Geometry: see drawing. Coordinates: mm, zero at the bounding-box minimum. A direction names the side the tool comes from. Give positions to 0.01 mm unless a question says otherwise; leave off trailing zeros. Order: outer loops, then holes, each group sorted by start corner. A loop starts at its lowest first (then second) coordinate and runs counter-clockwise, first axis right, second up. Notation, with made-up numbers: (-26, 27) - (-6, 27) arc R22 ccw to (-6, 58) - close; hole circle Ø4 at (25.25, 54.25). An arc over 180 degrees is marked (long way). Write item = value, one per line. Start each with the question number.
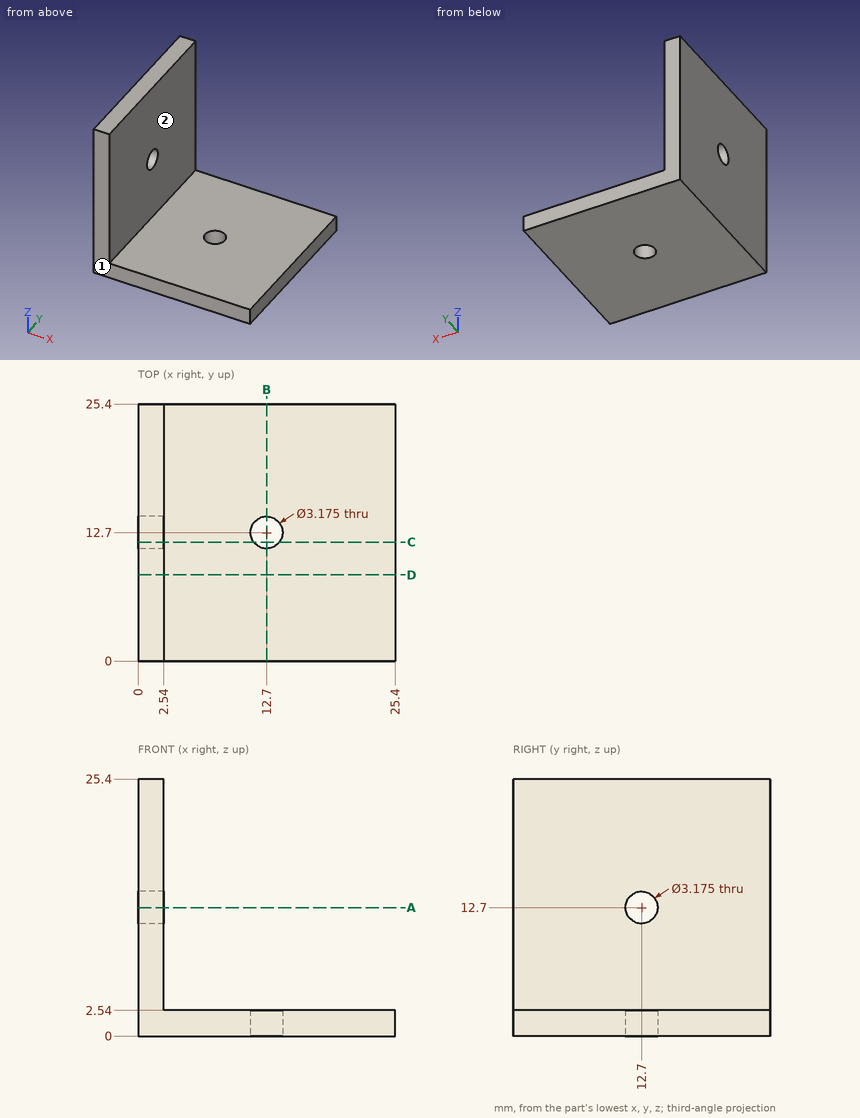
Q1. Section D-D, the plane y = 8.5. Return the cut outline in (x, z), then the cut area to 3 significant figures.
Q2. Section C-C, the plane y = 11.75. Return the cut outline in (x, z), then the cut area to 3 significant figures.
Q3. Set-up query: the marked faces 1 and 2. Return all of +Z, -Z, +X, -X, +Y, -Y with unobstructed straight access to the full face (end or side cutting, diameter ignored); none if empty.
Q4. Section A-A, the plane z = 12.7. Return the cut outline in (x, y).
Q5. Section B-B, the plane x = 12.7. Return the cut outline in (y, z).
Q6. Contact query for a flat-ended pin moving along its axis: pin 1 (8 mm diameter, centred on y = 6, z = 21.5, fed in from +X). Output: stop coordinate, or through.
Q7. Material intervals for line 1 along X through (y, z) = (8, 12.25); line 2 along Y through (x, z) = (12.7, 2), sorted ascending. Write a range as from..to.
The answers:
q1.outline = (0, 0) - (25.4, 0) - (25.4, 2.54) - (2.54, 2.54) - (2.54, 25.4) - (0, 25.4) - close
q1.area = 123 mm²
q2.outline = (0, 0) - (11.43, 0) - (11.43, 2.54) - (2.54, 2.54) - (2.54, 11.43) - (0, 11.43) - close; (0, 13.97) - (2.54, 13.97) - (2.54, 25.4) - (0, 25.4) - close; (13.97, 0) - (25.4, 0) - (25.4, 2.54) - (13.97, 2.54) - close
q2.area = 110 mm²
q3.face_1 = +Z, -Z, +X, -X, -Y
q3.face_2 = +Z, +X, +Y, -Y
q4.outline = (0, 0) - (2.54, 0) - (2.54, 11.11) - (0, 11.11) - close; (0, 14.29) - (2.54, 14.29) - (2.54, 25.4) - (0, 25.4) - close
q5.outline = (0, 0) - (11.11, 0) - (11.11, 2.54) - (0, 2.54) - close; (14.29, 0) - (25.4, 0) - (25.4, 2.54) - (14.29, 2.54) - close
q6.pin_1 = 2.54
q7.line_1 = 0..2.54
q7.line_2 = 0..11.11, 14.29..25.4
